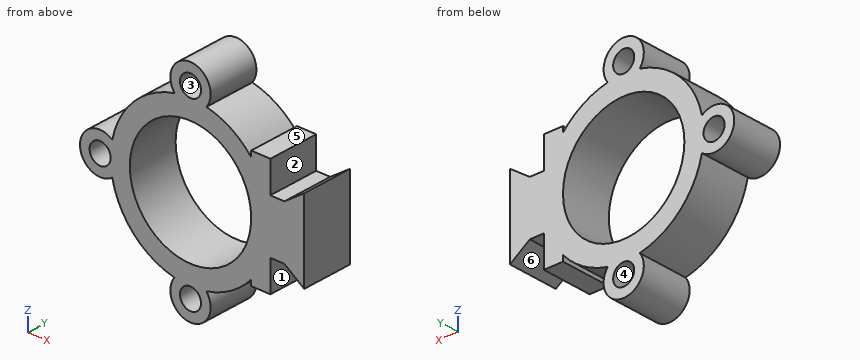
Autodesk Inventor part; units mm, degrees
ref_plane "YZ Plane" through (0, 0, 0) normal (1, 0, 0) x (0, 1, 0)
ref_plane "XZ Plane" through (0, 0, 0) normal (0, 1, 0) x (-1, 0, 0)
ref_plane "XY Plane" through (0, 0, 0) normal (0, 0, 1) x (1, 0, 0)
sketch "Boceto1" plane through (0, 0, 0) normal (0, 1, 0) x (-1, 0, 0)
  line L0 (0, 6.35) -> (0, -6.35)
  line L1 (3.1, 4.15) -> (3.1, -4.15)
  line L2 (0, 6.35) -> (3.1, 4.15)
  line L3 (3.1, -4.15) -> (0, -6.35)
  line L4 (3.1, 4.15) -> (5.3, 4.15)
  line L5 (-4.6452, 0) -> (17.8, 0) construction
  line L6 (3.1, -4.15) -> (5.3, -4.15)
  line L7 (5.3, 9) -> (5.3, -9)
  line L8 (5.3, 9) -> (8.3, 9)
  line L9 (8.3, 9) -> (8.3, -9)
  line L10 (8.3, -9) -> (5.3, -9)
  line L11 (5.3, -9) -> (5.3, 9)
  circle A0 centre (17.8, 0) radius 9.5
  circle A1 centre (17.8, 0) radius 12.5
  circle A2 centre (31.95, 0) radius 1.65
  circle A3 centre (31.95, 0) radius 3.15
  circle A4 centre (17.8, 14.15) radius 3.15
  circle A5 centre (17.8, 14.15) radius 1.65
  circle A6 centre (17.8, -14.15) radius 3.15
  circle A7 centre (17.8, -14.15) radius 1.65
  point P0 (0, 0)
  point P1 (0, 0)
  point P2 (3.1, 0)
  point P3 (5.3, 0)
  point P4 (5.3, 0)
  point P5 (30.3, 0)
  point P6 (17.8, -12.5)
  point P7 (17.8, 12.5)
  point P8 (30.0456, 2.5091)
  point P9 (20.3091, 12.2456)
  point P10 (15.2909, 12.2456)
  point P11 (8.3, 8.124)
  point P12 (8.3, -8.124)
  point P13 (15.2909, -12.2456)
  point P14 (20.3091, -12.2456)
  point P15 (30.0456, -2.5091)
  dimension "d0" = 12.7
  dimension "d1" = 8.3
  dimension "d2" = 3.1
  dimension "d3" = 2.2
  dimension "d4" = 18
  dimension "d5" = 3
  dimension "d6" = 19
  dimension "d7" = 25
  dimension "d8" = 3.3
  dimension "d9" = 6.3
  dimension "d12" = 90
  dimension "d16" = 90
extrude "Extrusión1" add sketch "Boceto1" along normal blind 8
properties part number "acople_v2_3DPrint"
Verification items for the finished model (mm, model axes). Face numbers are marked on the shaded views. A direction names the side the tool comes from. Give positions to 0.01 mm unless a question says otherwise; leave off trailing zeros. Write each loop counter-clockwise with the first axis right and the second up, starting at its lowest first coordinate (ties: lowest second). Pieces come first, ordered by that corner, then holes. Notation, with made-up numbers: M -39,54 L 5,54 A10 ccw 5,59 Z; hole C 53,56.5 d11. An arc over 180 degrees is marked long. One line per question, with ' | ' between items.
1) Section check A-A on z = 0. Enter the section's corners in (x, y), plus the area to 3 significant figures.
Result:
outline: M -35.1,0 L -33.6,0 L -33.6,8 L -35.1,8 Z; M -30.3,0 L -27.3,0 L -27.3,8 L -30.3,8 Z; M -8.3,0 L 0,0 L 0,8 L -8.3,8 Z | area: 102 mm2
2) Mould release check, pull along Z, two halves, no side actions. Record for the marked faces 4, 5 and 6: released by +Z, released by -Z, zero draft, split by the parting line, or undercut.
Result:
face 4: undercut | face 5: released by +Z | face 6: released by -Z
3) Section check D-D on x = -31.95. Enter the section's corners in (y, z), plus the area to 3 significant figures.
Result:
outline: M 0,-3.15 L 8,-3.15 L 8,-1.65 L 0,-1.65 Z; M 0,1.65 L 8,1.65 L 8,3.15 L 0,3.15 Z | area: 24.0 mm2
4) Thickness scan on line 1 along X through (y, z) = (5.5, 0); line 2 along X through (y, z) = (2.25, 14.15); line 3 along Z through (x, y) = (-17.8, 3.5). Record the ranges inside material, lowest first. Write a range as [from, to].
Result:
line 1: x = [-35.1, -33.6], [-30.3, -27.3], [-8.3, 0] | line 2: x = [-20.95, -19.45], [-16.15, -14.65] | line 3: z = [-17.3, -15.8], [-12.5, -9.5], [9.5, 12.5], [15.8, 17.3]
5) Section check B-B on x = -17.8. Enter the section's corners in (y, z).
Result:
outline: M 0,-17.3 L 8,-17.3 L 8,-15.8 L 0,-15.8 Z; M 0,-12.5 L 8,-12.5 L 8,-9.5 L 0,-9.5 Z; M 0,9.5 L 8,9.5 L 8,12.5 L 0,12.5 Z; M 0,15.8 L 8,15.8 L 8,17.3 L 0,17.3 Z
6) Section check C-C on y = 4.5. Enter the section's corners in (x, z), plus the area to 3 significant figures.
Result:
outline: M -30.05,-2.51 A12.5 ccw -20.31,-12.25 A3.15 ccw long -15.29,-12.25 A12.5 ccw -8.3,-8.12 L -8.3,-9 L -5.3,-9 L -5.3,-4.15 L -3.1,-4.15 L 0,-6.35 L 0,6.35 L -3.1,4.15 L -5.3,4.15 L -5.3,9 L -8.3,9 L -8.3,8.12 A12.5 ccw -15.29,12.25 A3.15 ccw long -20.31,12.25 A12.5 ccw -30.05,2.51 A3.15 ccw long Z; hole C -31.95,0 d3.3; hole C -17.8,0 d19; hole C -17.8,-14.15 d3.3; hole C -17.8,14.15 d3.3 | area: 331 mm2
7) Set-up check for the marked faces 1, 2 and 3: record each of +Z, -Z, +X, -X, +Y, -Y from which the full face is reachable in a straight line by a thin tool's end or side.
Result:
face 1: -Z, +Y, -Y | face 2: +Z, +Y, -Y | face 3: +Y, -Y
8) Gauge pin test, flat ends, axial feed: pin 1 Ø1.5 at (y, z) = (5.5, -6) entering from -X; pin 2 Ø3 at (x, z) = (-17.8, -14.15) entering from -Y; pin 3 Ø1.1 at (x, y) = (-4, 3) entering from -Z; pin 4 Ø0.7 at (x, y) = (-4, 3) entering from +Z. Record the tip position at first contact, or that the pin passes through.
Result:
pin 1: stops at x = -29.14 | pin 2: passes through | pin 3: stops at z = -4.15 | pin 4: stops at z = 4.15
